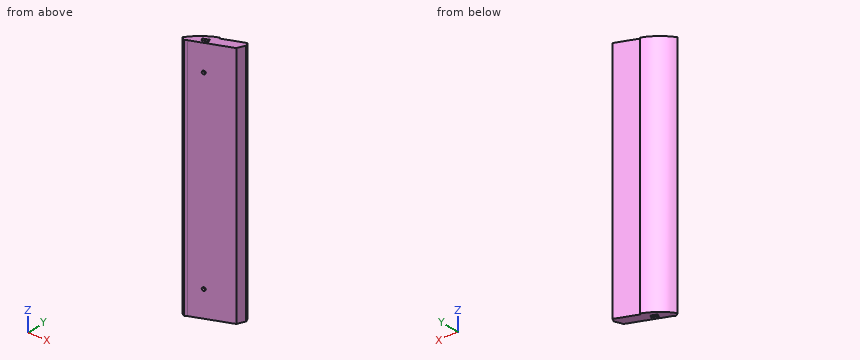
Autodesk Inventor part; units mm, degrees
ref_plane "Work Plane1" through (0, 0, 122.75) normal (0, 0, -1) x (-1, 0, 0)
ref_plane "YZ Plane" through (0, 0, 0) normal (1, 0, 0) x (0, 1, 0)
ref_plane "XZ Plane" through (0, 0, 0) normal (0, 1, 0) x (-1, 0, 0)
sketch "Sketch1" plane through (0, 0, 0) normal (0, 0, 1) x (1, 0, 0)
  line L0 (10, 0) -> (-1.5, 0)
  line L1 (10, 45.2667) -> (10, 0)
  arc A0 (13.0769, 49.8821) -> (10, 45.2667) centre (15, 45.2667) ccw
  line L2 (54.8615, 67.2923) -> (13.0769, 49.8821)
  line L3 (50.4385, 77.9077) -> (54.8615, 67.2923)
  line L4 (50.4385, 77.9077) -> (29.2692, 69.0872)
  arc A1 (29.2692, 69.0872) -> (-1.5, 22.9333) centre (48.5, 22.9333) ccw
  line L5 (-1.5, 0) -> (-1.5, 22.9333)
  line L6 (29.2692, 69.0872) -> (33.9692, 58.5872)
  line L7 (15, 45.2667) -> (6.8975, 50.6683)
  line L8 (29.2692, 69.0872) -> (50.4077, 77.8949)
  line L9 (50.4077, 77.8949) -> (52.5231, 72.8179)
  line L10 (52.5231, 72.8179) -> (49.2923, 64.9718)
  line L11 (29.8823, 67.7176) -> (50.9846, 76.5103)
  point P0 (0, 0)
  point P1 (10.8397, 48.0402)
  dimension "d2" = 22.9
  dimension "d3" = 5.5
  dimension "d4" = 45
  dimension "d5" = 1.5
extrude "Extrusion1" add sketch "Sketch1" along normal blind 245.5 contours L7 A1 L6 L2 A0 | L6 L11 L9 L10 L2
sketch "Sketch2" plane through (10.8397, 48.0402, 0) normal (-0.5547, -0.8321, 0) x (0.8321, -0.5547, 0)
  line L0 (-4.738, 0) -> (0, 0)
  line L1 (0, 0) -> (0, 245.5)
  line L2 (-4.738, 245.5) -> (0, 245.5)
  line L3 (-4.738, 0) -> (-4.738, 245.5)
  circle A0 centre (-2.238, 15) radius 1.25
  circle A1 centre (-2.238, 65) radius 1.25
  circle A2 centre (-2.238, 115) radius 1.25
  circle A3 centre (-2.238, 165) radius 1.25
  circle A4 centre (-2.238, 215) radius 1.25
  point P0 (17.6287, 0)
  dimension "d6" = 2.5
  dimension "d7" = 2.5
  dimension "d8" = 15
  dimension "d11" = 50
extrude "Extrusion2" cut sketch "Sketch2" against normal blind 3 contours A0 | A1 | A2 | A3 | A4
sketch "Sketch3" plane through (0, 0, 0) normal (0, 0, -1) x (-1, 0, 0)
  line L0 (-13.0769, 49.8821) -> (-49.2923, 64.9718)
  line L1 (-26.6245, 58.7769) -> (-21.086, 56.4692)
  line L2 (-21.086, 56.4692) -> (-19.9322, 59.2384)
  line L3 (-19.9322, 59.2384) -> (-25.4706, 61.5461)
  line L4 (-25.4706, 61.5461) -> (-26.6245, 58.7769)
  arc A0 (-10.8397, 48.0402) -> (-13.0769, 49.8821) centre (-15, 45.2667) ccw
  line L5 (-6.8975, 50.6683) -> (-10.8397, 48.0402)
  arc A1 (-6.8975, 50.6683) -> (-29.2692, 69.0872) centre (-48.5, 22.9333) ccw
  line L6 (-29.8823, 67.7176) -> (-29.2692, 69.0872)
  line L7 (-50.9846, 76.5103) -> (-29.8823, 67.7176)
  line L8 (-52.5231, 72.8179) -> (-50.9846, 76.5103)
  line L9 (-49.2923, 64.9718) -> (-52.5231, 72.8179)
  line L10 (-13.0769, 49.8821) -> (-49.2923, 64.9718)
  point P0 (0, 0)
  dimension "d20" = 6
  dimension "d21" = 3
  dimension "d22" = 3
  dimension "d32" = 12.7
extrude "Extrusion3" cut sketch "Sketch3" against normal blind 30 contours L4 L3 L2 L1
sketch "Sketch4" plane through (49.2923, 64.9718, 0) normal (0.3846, -0.9231, 0) x (0.9231, 0.3846, 0)
  line L0 (-29.3068, 0) -> (-23.3068, 0)
  line L1 (-29.3068, 0) -> (-29.3068, 30)
  line L2 (-29.3068, 30) -> (-23.3068, 30)
  line L3 (-23.3068, 0) -> (-23.3068, 30)
  circle A0 centre (-26.3068, 26.4) radius 1.65
  line L4 (-26.3068, 29.7486) -> (-23.4068, 28.0743)
  line L5 (-23.4068, 28.0743) -> (-23.4068, 24.7257)
  line L6 (-23.4068, 24.7257) -> (-26.3068, 23.0514)
  line L7 (-26.3068, 23.0514) -> (-29.2068, 24.7257)
  line L8 (-29.2068, 24.7257) -> (-29.2068, 28.0743)
  line L9 (-29.2068, 28.0743) -> (-26.3068, 29.7486)
  point P0 (-70.4897, 0)
  point P1 (-26.3068, 30)
  dimension "d26" = 3.3
  dimension "d27" = 3.6
  dimension "d28" = 5.8
extrude "Extrusion4" cut sketch "Sketch4" against normal blind 7 contours A0
ref_plane "Work Plane1" through (0, 0, 122.75) normal (0, 0, -1) x (-1, 0, 0)
mirror "Mirror1" about plane through (0, 0, 122.75) normal (0, 0, -1) of "Extrusion4", "Extrusion3"
properties part number "ESQUINA_REDONDEADA_R50"
For this review, take the finished solid that the model builds, in its own axes (mm). Give positions to 0.01 mm unless a question says otherwise; leave off trailing zeros. Order: outer loops, then holes, each group sorted by start corner. A loop starts at its lowest first (then second) coordinate and runs counter-clockwise, first axis right, second up. Notation, with made-up numbers: (45, 72.25) -> (87, 72.25) arc R28 cw to (87, 99.25) -> close; hole circle Ø11 at (63.25, 54.5). An arc over 180 degrees is marked (long way). Write item = value, one per line.
1) Insertion check: pin 1 (8 mm diameter, centred on y = 62, z = 94.5, fed in from +X); pin 2 (1 mm diameter, centred on y = 72, z = 26.5, fed in from +X); pin 3 (1 mm diameter, centred on x = 19, z = 220, fed in from +Y). Each pin has a flat end and moves straight along its axis. Give the tip position at first contact, or say it passes through.
Findings:
pin_1 = 49.72
pin_2 = 52.39
pin_3 = 63.66
2) We need section B-B, the plane z = 199. Give the boundary of the cut face in (x, y).
Findings:
outline = (6.9, 50.67) -> (10.84, 48.04) arc R5 cw to (13.08, 49.88) -> (49.29, 64.97) -> (52.52, 72.82) -> (50.98, 76.51) -> (29.88, 67.72) -> (29.27, 69.09) arc R50 ccw to start
3) We need section A-A, the plane z = 22. Give the boundary of the cut face in (x, y).
Findings:
outline = (6.9, 50.67) -> (10.84, 48.04) arc R5 cw to (13.08, 49.88) -> (49.29, 64.97) -> (52.52, 72.82) -> (50.98, 76.51) -> (29.88, 67.72) -> (29.27, 69.09) arc R50 ccw to start; hole (19.93, 59.24) -> (21.09, 56.47) -> (26.62, 58.78) -> (25.47, 61.55) -> close
4) To check wall thickness, follow L1, parallel to Y at x = 25, z = 20; L2, parallel to X at y = 60, z = 219.5; L3, parallel to X at y = 59, z = 234.5. State the ranges of each line that lie inside material, in increasing order. Write a range as from..to.
Findings:
L1 = 54.85..58.1, 61.35..67.07
L2 = 14.94..21.13, 26.11..37.36
L3 = 13.87..20.03, 26.53..34.96
5) We need section C-C, the plane x = 40.5. Give the boundary of the cut face in (y, z), and give its area (3 significant figures).
Findings:
outline = (61.31, 0) -> (72.14, 0) -> (72.14, 245.5) -> (61.31, 245.5) -> close
area = 2,660 mm^2
